```python
from build123d import *

# Parameters (mm, degrees)
BOSS_EXTRUDE1_DEPTH = 46
CUT_EXTRUDE1_DEPTH  = 77.26270386
SKETCH3_R           = 6
CUT_EXTRUDE2_DEPTH  = 77.26270386
SKETCH5_R           = 3
CUT_EXTRUDE3_DEPTH  = 82.437092286
SKETCH6_R           = 4
CUT_EXTRUDE4_DEPTH  = 16
CUT_EXTRUDE5_DEPTH  = 77.262703957


with BuildPart() as part:
    # Sketch1 → Boss-Extrude1 (new body)
    with BuildSketch(Plane.XY):
        with BuildLine():
            Line((22.627416998, 0), (28, 0))
            Line((28, 0), (28, 16))
            Line((28, 16), (54, 16))
            Line((54, 16), (54, 28))
            Line((54, 28), (31.749015733, 28))
            ThreePointArc((31.749015733, 28), (0, 40), (-31.749015733, 28))
            Line((-31.749015733, 28), (-54, 28))
            Line((-54, 28), (-54, 16.005791269))
            Line((-54, 16.005791269), (-28, 16.005791269))
            Line((-28, 16.005791269), (-28, 0))
            Line((-28, 0), (-22.627416998, 0))
            ThreePointArc((-22.627416998, 0), (0, 16), (22.627416998, 0))
        make_face()
    extrude(amount=BOSS_EXTRUDE1_DEPTH)

    # Sketch2 → Cut-Extrude1 (cut, through all)
    with BuildSketch(Plane(origin=(0, 28, 0), x_dir=(1, 0, 0), z_dir=(0, 1, 0))):
        with BuildLine():
            Line((54, -46), (54, -23))
            ThreePointArc((54, -23), (52.698550436, -34.784005345), (48.856934001, -46))
            Line((48.856934001, -46), (54, -46))
        make_face()
        with BuildLine():
            Line((54, 0), (48.856934001, 0))
            ThreePointArc((48.856934001, 0), (52.698550436, -11.215994655), (54, -23))
            Line((54, -23), (54, 0))
        make_face()
        with BuildLine():
            ThreePointArc((-54, -23.000000162), (-52.698550453, -11.215994734), (-48.856934001, 0))
            Line((-48.856934001, 0), (-54, 0))
            Line((-54, 0), (-54, -23.000000162))
        make_face()
        with BuildLine():
            ThreePointArc((-48.856934001, -46), (-52.698550418, -34.784005424), (-54, -23.000000162))
            Line((-54, -23.000000162), (-54, -46))
            Line((-54, -46), (-48.856934001, -46))
        make_face()
    extrude(amount=-CUT_EXTRUDE1_DEPTH, mode=Mode.SUBTRACT)

    # Sketch3 → Cut-Extrude2 (cut, through all)
    with BuildSketch(Plane(origin=(0, 28, 0), x_dir=(1, 0, 0), z_dir=(0, 1, 0))):
        with Locations(Location((39, -23, 0), (0, 0, 180))):
            Circle(SKETCH3_R)
        with Locations(Location((-39, -23, 0), (0, 0, 270))):
            Circle(SKETCH3_R)
    extrude(amount=-CUT_EXTRUDE2_DEPTH, mode=Mode.SUBTRACT)

    # Sketch5 → Cut-Extrude3 (cut, through all)
    with BuildSketch(Plane(origin=(0, 40, 0), x_dir=(1, 0, 0), z_dir=(0, 1, 0))):
        with Locations(Location((0, -23, 0), (0, 0, 270))):
            Circle(SKETCH5_R)
    extrude(amount=-CUT_EXTRUDE3_DEPTH, mode=Mode.SUBTRACT)

    # Sketch6 → Cut-Extrude4 (cut)
    with BuildSketch(Plane(origin=(0, 40, 0), x_dir=(1, 0, 0), z_dir=(0, 1, 0))):
        with Locations(Location((0, -23, 0), (0, 0, 270))):
            Circle(SKETCH6_R)
    extrude(amount=-CUT_EXTRUDE4_DEPTH, mode=Mode.SUBTRACT)

    # Sketch7 → Cut-Extrude5 (cut, through all)
    with BuildSketch(Plane(origin=(0, 28, 0), x_dir=(1, 0, 0), z_dir=(0, 1, 0))):
        with BuildLine():
            ThreePointArc((-31.749015733, -7.623939804), (-22, -23), (-31.749015733, -38.376060196))
            Line((-31.749015733, -38.376060196), (-31.749015733, -7.623939804))
        make_face()
        with BuildLine():
            Line((31.749015733, -38.376060196), (31.749015733, -7.623939804))
            ThreePointArc((31.749015733, -7.623939804), (22, -23), (31.749015733, -38.376060196))
        make_face()
    extrude(amount=CUT_EXTRUDE5_DEPTH, mode=Mode.SUBTRACT)


solid = part.part
```
Read the model definition and answer for the solid it produces. Units are mm, in the model's axes. A direction names the side the tool comes from. Give positions to 0.01 mm unless a question says otherwise; leave off trailing zeros. Loops run counter-clockwise (first coordinate to the right, second up) from the corner with the lowest first, then second, coordinate; pieces in that order, holes last.
Item 1: The part is cut by section B-B (z = 14.5). Write down the section's boundary in (x, y).
Item 2: The mould has two halves that part along X. Classify faces 5 (the flat face through (3, 24, 24)), 6 (the flat face through (-28, 8, 23)), 7 (the flat face through (25, 0, 23)), 8 (the cylindrical face through (0, 20, 20)): released by +X, released by -X, zero draft, split by the parting line, or undercut.
Item 3: The part is cut by section C-C (x = -39). Write down the section's boundary in (y, z), and give its area (3 significant figures).
Item 4: The part is cut by section A-A (x = 39). Write down the section's boundary in (y, z), and give its area (3 significant figures).
Item 5: For faces 1 (the cylindrical face through (-22, 31, 23)), 2 (the flat face through (44, 16, 18)), 3 (the flat face through (-44, 16.006, 28)), 4 (the cylindrical face through (22, 31, 23)), determine the directions among +Z, -Z, +X, -X, +Y, -Y from which every point of the face is accessible in a straight line to the end or side of a thin tool.
Item 6: The part is cut by section D-D (x = 0). Write down the section's boundary in (y, z), and give its area (3 significant figures).
Item 7: Each of these flat-tipped pins is pushed along its axis until it touches: pin 1 Ø8 at (y, z) = (31.5, 32.5) entering from -X; pin 2 Ø8 at (x, y) = (-41.5, 13) entering from +Z; pin 3 Ø1.5 at (y, z) = (19, 5.5) entering from -X; pin 4 Ø13 at (x, z) = (-40, 24.5) entering from -Y. Where does it stop, or does it pass through?
Item 8: Find the intervals of material crossed by line 1 along Z through (x, y) = (0, 35.25); line 2 along Z through (x, y) = (39, 21.5); line 3 along X through (y, z) = (31, 40.5), in increasing order.
Taken from the geometry:
1. outline: (-53.33, 16.01) - (-28, 16.01) - (-28, 0) - (-22.63, 0) arc R24 cw to (22.63, 0) - (28, 0) - (28, 16) - (53.33, 16) - (53.33, 28) - (24.28, 28) - (24.28, 33.41) arc R48 ccw to (-24.28, 33.41) - (-24.28, 28) - (-53.33, 28) - close
2. face 5: undercut
2. face 6: released by -X
2. face 7: zero draft
2. face 8: undercut
3. outline: (16.01, 0) - (28, 0) - (28, 17) - (16.01, 17) - close; (16.01, 29) - (28, 29) - (28, 46) - (16.01, 46) - close
3. area: 408 mm2
4. outline: (16, 0) - (28, 0) - (28, 17) - (16, 17) - close; (16, 29) - (28, 29) - (28, 46) - (16, 46) - close
4. area: 408 mm2
5. face 1: -X, +Y
5. face 2: +Z, -Z, +X, -Y
5. face 3: +Z, -Z, -X, -Y
5. face 4: +X, +Y
6. outline: (16, 0) - (40, 0) - (40, 19) - (24, 19) - (24, 20) - (16, 20) - close; (16, 26) - (24, 26) - (24, 27) - (40, 27) - (40, 46) - (16, 46) - close
6. area: 928 mm2
7. pin 1: stops at x = -53.47
7. pin 2: stops at z = 46
7. pin 3: stops at x = -51.34
7. pin 4: stops at y = 16.01
8. line 1: z = 0 to 19, 27 to 46
8. line 2: z = 0 to 17, 29 to 46
8. line 3: x = -27.98 to 27.98
